Could you check a few things on this model? Use its own coordinates, in mm. Face numbers are marked on the shaded views. A direction names the side the tool comes from. Give positions to 0.01 mm unless a question says otherwise; leave off trailing zeros. Order: outer loops, then holes, each group sorted by start corner. A loop starts at its lowest first (then second) coordinate and runs counter-clockwise, first axis right, second up.
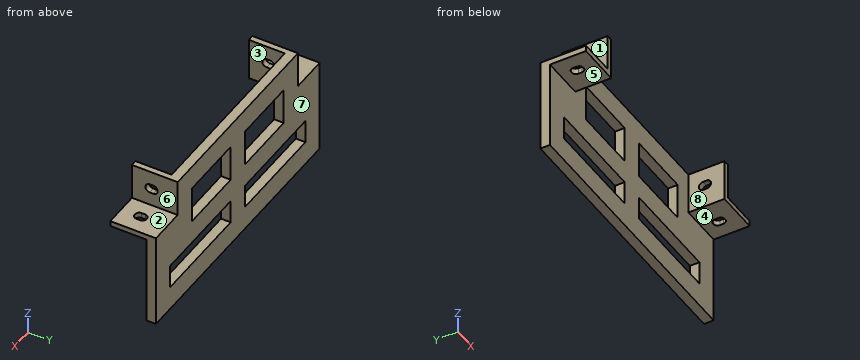
Solid Edge part; units mm, degrees
sketch "Sketch1" plane through (0, 0, 0) normal (0, -1, 0) x (1, 0, 0)
  line L0 (-10, 50.25) -> (-64.5, 50.25)
  line L1 (-64.5, 50.25) -> (-64.5, 19.75)
  line L2 (-64.5, 19.75) -> (-10, 19.75)
  line L3 (-10, 50.25) -> (-10, 19.75)
  line L4 (-10, 0) -> (-95, 0)
  line L5 (-95, 0) -> (-95, -19.75)
  line L6 (-95, -19.75) -> (-10, -19.75)
  line L7 (-10, 0) -> (-10, -19.75)
  line L8 (95, -19.75) -> (95, 0)
  line L9 (95, 0) -> (10, 0)
  line L10 (10, -19.75) -> (10, 0)
  line L11 (10, -19.75) -> (95, -19.75)
  line L12 (-84.5, 39.75) -> (-115, 39.75)
  line L13 (-115, 39.75) -> (-115, -39.75)
  line L14 (-115, -39.75) -> (115, -39.75)
  line L15 (115, -39.75) -> (115, 39.75)
  line L16 (115, 39.75) -> (84.5, 39.75)
  line L17 (84.5, 39.75) -> (84.5, 70.25)
  line L18 (84.5, 70.25) -> (-84.5, 70.25)
  line L19 (-84.5, 70.25) -> (-84.5, 39.75)
  line L20 (10, 19.75) -> (64.5, 19.75)
  line L21 (64.5, 19.75) -> (64.5, 50.25)
  line L22 (64.5, 50.25) -> (10, 50.25)
  line L23 (10, 19.75) -> (10, 50.25)
extrude "Protrusion1" add sketch "Sketch1" along normal blind 8
sketch "Sketch2" plane through (0, -8, 15.25) normal (0, -1, 0) x (1, 0, 0)
  line L0 (-115, 24.5) -> (-115, 19.5)
  line L1 (-115, 19.5) -> (-79.5, 19.5)
  line L2 (-79.5, 19.5) -> (-79.5, 55)
  line L3 (-84.5, 55) -> (-79.5, 55)
  line L4 (-84.5, 55) -> (-84.5, 24.5)
  line L5 (-84.5, 24.5) -> (-115, 24.5)
  line L6 (115, 19.9501) -> (79.5, 19.9501)
  line L7 (79.5, 19.9501) -> (79.5, 55)
  line L8 (84.5, 55) -> (79.5, 55)
  line L9 (84.5, 55) -> (84.5, 24.5)
  line L10 (84.5, 24.5) -> (115, 24.5)
  line L11 (115, 24.5) -> (115, 19.9501)
extrude "Protrusion2" add sketch "Sketch2" along normal blind 30
sketch "Sketch3" plane through (-97.25, -23, 34.75) normal (0, 0, -1) x (1, 0, 0)
  arc A0 (-2, -6.25) -> (1.5, -2.75) centre (-2, -2.75) ccw
  line L0 (1.5, -2.75) -> (1.5, 0.25)
  arc A1 (1.5, 0.25) -> (-2, 3.75) centre (-2, 0.25) ccw
  line L1 (-2, 3.75) -> (-2.5, 3.75)
  arc A2 (-2.5, 3.75) -> (-6, 0.25) centre (-2.5, 0.25) ccw
  line L2 (-6, 0.25) -> (-6, -2.75)
  arc A3 (-6, -2.75) -> (-2.5, -6.25) centre (-2.5, -2.75) ccw
  line L3 (-2.5, -6.25) -> (-2, -6.25)
extrude "Cutout1" cut sketch "Sketch3" against normal blind 20
sketch "Sketch4" plane through (97.25, -23, 35.2001) normal (0, 0, -1) x (1, 0, 0)
  arc A0 (2.5, -6.25) -> (6, -2.75) centre (2.5, -2.75) ccw
  line L0 (6, -2.75) -> (6, 0.25)
  arc A1 (6, 0.25) -> (2.5, 3.75) centre (2.5, 0.25) ccw
  line L1 (2.5, 3.75) -> (2, 3.75)
  arc A2 (2, 3.75) -> (-1.5, 0.25) centre (2, 0.25) ccw
  line L2 (-1.5, 0.25) -> (-1.5, -2.75)
  arc A3 (2, -6.25) -> (-1.5, -2.75) centre (2, -2.75) cw
  line L3 (2, -6.25) -> (2.5, -6.25)
extrude "Cutout2" cut sketch "Sketch4" against normal blind 40
sketch "Sketch5" plane through (-84.5, -19, 55) normal (-1, 0, 0) x (0, 0, -1)
  arc A0 (0.5, -2.25) -> (4, 1.25) centre (0.5, 1.25) ccw
  line L0 (4, 1.25) -> (4, 4.25)
  arc A1 (4, 4.25) -> (0.5, 7.75) centre (0.5, 4.25) ccw
  line L1 (0.5, 7.75) -> (0, 7.75)
  arc A2 (0, 7.75) -> (-3.5, 4.25) centre (0, 4.25) ccw
  line L2 (-3.5, 4.25) -> (-3.5, 1.25)
  arc A3 (0, -2.25) -> (-3.5, 1.25) centre (0, 1.25) cw
  line L3 (0, -2.25) -> (0.5, -2.25)
extrude "Cutout3" cut sketch "Sketch5" against normal blind 200
Item 1: For the marked faces 1, 2, 3, 4 and 5, which set-ups out of +Z, -Z, +X, -X, +Y, -Y let a thin tool reach every point of the face, with its end or its side?
Findings:
face 1: +Z, -X, +Y, -Y
face 2: +Z, +X, +Y, -Y
face 3: +Z, -Z, -Y
face 4: -Z, +X, -Y
face 5: -Z, +X, -X, -Y
Item 2: Imagine slicing it at C-C on x = -75. List the corners of the cut face in (y, z) for me, then the cut area to 3 significant figures.
Findings:
outline: (-8, -39.75) - (0, -39.75) - (0, -19.75) - (-8, -19.75) - close; (-8, 0) - (0, 0) - (0, 70.25) - (-8, 70.25) - close
area: 722 mm2
Item 3: Imagine slicing it at D-D on x = -20.5. List the corners of the cut face in (y, z) for me, then the cut area to 3 significant figures.
Findings:
outline: (-8, -39.75) - (0, -39.75) - (0, -19.75) - (-8, -19.75) - close; (-8, 0) - (0, 0) - (0, 19.75) - (-8, 19.75) - close; (-8, 50.25) - (0, 50.25) - (0, 70.25) - (-8, 70.25) - close
area: 478 mm2
Item 4: We'd pull the mould along X, two halves only. Please class the marked faces 6, 7 and 8: +X half, -X half, draft (parallel to the pull), parting line (faces both ways), or undercut.
Findings:
face 6: +X half
face 7: draft
face 8: undercut
Item 5: Imagine slicing it at B-B on y = -30. List the corners of the cut face in (x, z) for me.
Findings:
outline: (-115, 34.75) - (-79.5, 34.75) - (-79.5, 70.25) - (-84.5, 70.25) - (-84.5, 39.75) - (-115, 39.75) - close; (79.5, 35.2) - (115, 35.2) - (115, 39.75) - (84.5, 39.75) - (84.5, 70.25) - (79.5, 70.25) - close
Item 6: For pin 1 (15 mm diameter, centred on x = 99, y = -13, fed in from +Z); pin 2 (8 mm diameter, centred on x = 57, z = 59, fed in from -Y), each with a flat end and sliding along its axis, tell me the tip position at first contact or that it passes through.
Findings:
pin 1: stops at z = 39.75
pin 2: stops at y = -8
Item 7: Imagine slicing it at A-A on z = 45. List the corners of the cut face in (x, y) for me.
Findings:
outline: (-84.5, -38) - (-79.5, -38) - (-79.5, -8) - (-64.5, -8) - (-64.5, 0) - (-84.5, 0) - close; (-10, -8) - (10, -8) - (10, 0) - (-10, 0) - close; (64.5, -8) - (79.5, -8) - (79.5, -38) - (84.5, -38) - (84.5, 0) - (64.5, 0) - close
Item 8: Please list where these lines run through material, in increasing order: line 1 along Z through (x, y) = (-36, -4); line 2 along X through (y, z) = (-2, -5); line 3 along X through (y, z) = (-21, 43).
Findings:
line 1: z = -39.75 to -19.75, 0 to 19.75, 50.25 to 70.25
line 2: x = -115 to -95, -10 to 10, 95 to 115
line 3: x = -84.5 to -79.5, 79.5 to 84.5
